The model under review builds one solid part; all positions refer to its coordinate system, in mm. A direction names the side the tool comes from. Round coordinates to 2 decimals unless told otherwise and drop trailing zeros. Loops run counter-clockwise (first coordinate to the right, second up) from the corner with the lowest first, then second, coordinate; pieces in that order, holes last. Notation, with made-up numbers: M -26,-11 L 23,-11 A23 cw 23,6 Z; hole C -39.75,-34 d7. An arc over 180 degrees is marked long. Return JSON: item names as keys, results as strings. Group by question number.
Q1. Consider section C-C (x = 15.5). State the section outline as (y, z) points (3 decimals).
Q2. Consider section D-D (y = -28). Count the separate pieces of the cut face and the enclosed holes in it, and give its area (3 significant figures).
Q3. Draft analysis for pull direction Y (two halves, no side actions). For faces 1 (the face through (0, -5, -54)), 2 (the face through (15.697, -55.431, 42.503)), 3 (the face through (16, -9.525, 24)), state which applies: pulls with the +Y half, pulls with the -Y half, needs draft (parallel to the pull), parting line crosses it, or undercut.
Q4. Consider section A-A (z = 0). State the section outline as (x, y) points (3 decimals), and give its area (3 significant figures).
Q5. To check wall thickness, follow line 1 along Y through (x, z) = (23, 18) (3 decimals); line 2 along Y through (x, z) = (24.5, 17) (3 decimals); line 3 along Z through (x, y) = (7, 19) (3 decimals). State the ranges of each line that lie inside material, in increasing order.
Q6. Clearance check with flat-ended pins moving along their axes: pin 1 Ø15 at (x, y) = (14.5, -29) entering from -Z; pin 2 Ø5.5 at (x, y) = (11.5, 27) entering from -Z; pin 3 Ø5 at (x, z) = (11.5, -40) entering from -Y. State where each tip first meets the part, or that it passes through.
Q7. For faces 4 (the face through (27.01, -49.592, 11.012)), 5 (the face through (16.01, 10.43, 10.48)), 6 (the face through (31.75, -5, -54)), list the 3-axis set-ups (+Z, -Z, +X, -X, +Y, -Y) from which the entire face can be reached by the end or side of a thin tool; tool diameter is ignored.
Autodesk Inventor part; units mm, degrees
ref_plane "YZ Plane" through (0, 0, 0) normal (1, 0, 0) x (0, 1, 0)
ref_plane "XZ Plane" through (0, 0, 0) normal (0, 1, 0) x (-1, 0, 0)
ref_plane "XY Plane" through (0, 0, 0) normal (0, 0, 1) x (1, 0, 0)
sketch "Sketch1" plane through (0, 0, 0) normal (1, 0, 0) x (0, 1, 0)
  point P0 (0, 0)
sketch "Sketch2" plane through (0, 0, 0) normal (1, 0, 0) x (0, 1, 0)
  circle A0 centre (0, 0) radius 69.85
  dimension "d0" = 139.7
extrude "Extrusion1" add sketch "Sketch2" along normal blind 31.75
sketch "Sketch3" plane through (0, 0, 0) normal (-1, 0, 0) x (0, 0, 1)
  circle A0 centre (0, 0) radius 50.8
  dimension "d3" = 101.6
extrude "Extrusion2" cut sketch "Sketch3" against normal blind 6.35
sketch "Sketch4" plane through (31.75, 0, 0) normal (1, 0, 0) x (0, 0, -1)
  circle A0 centre (0, 0) radius 50.8
  dimension "d6" = 101.6
extrude "Extrusion3" cut sketch "Sketch4" against normal blind 6.35
sketch "Sketch5" plane through (6.35, 0, 0) normal (-1, 0, 0) x (0, 0, 1)
  circle A0 centre (0, 0) radius 9.525
  line L0 (9.525, 0) -> (9.525, 40.1609)
  circle A1 centre (0, 0) radius 50.8
  line L1 (9.525, -9.525) -> (9.525, -40.1609)
  line L2 (-9.525, 9.525) -> (-40.1609, 9.525)
  line L3 (9.525, 9.525) -> (40.1609, 9.525)
  line L4 (-9.525, 9.525) -> (-9.525, 40.1609)
  line L5 (-9.525, -9.525) -> (-9.525, -40.1609)
  line L6 (-9.525, -9.525) -> (-40.1609, -9.525)
  line L7 (9.525, -9.525) -> (40.1609, -9.525)
  arc A2 (9.525, -40.1609) -> (40.1609, -9.525) centre (0, 0) ccw
  arc A3 (40.1609, 9.525) -> (9.525, 40.1609) centre (0, 0) ccw
  arc A4 (-9.525, 40.1609) -> (-40.1609, 9.525) centre (0, 0) ccw
  arc A5 (-40.1609, -9.525) -> (-9.525, -40.1609) centre (0, 0) ccw
sketch "Sketch6" plane through (6.35, 0, 0) normal (-1, 0, 0) x (0, 0, 1)
  point P0 (0, 0)
sketch "Sketch7" plane through (6.35, 0, 0) normal (-1, 0, 0) x (0, 0, 1)
  point P0 (0, 0)
extrude "Extrusion4" cut sketch "Sketch5" against normal through all contours A0 | L0 A3 L3 | L7 A2 L1 | L2 A4 L4 | L5 A5 L6
fillet "Fillet1" radius 3.175 12 edges at (15.875, 9.525, -9.525) (15.875, 9.525, 9.525) (15.875, -9.525, 9.525) (15.875, 40.1609, 9.525) (15.875, 9.525, 40.1609) (15.875, -40.1609, 9.525) (15.875, 9.525, -40.1609) (15.875, -9.525, -9.525) (15.875, -9.525, -40.1609) (15.875, -40.1609, -9.525) (15.875, -9.525, 40.1609) (15.875, 40.1609, -9.525)
fillet "Fillet2" radius 3.175 4 edges at (0, -69.85, 0) (0, 0, -50.8) (31.75, -69.85, 0) (31.75, 0, 50.8)
sketch "Sketch8" plane through (31.75, 0, 0) normal (1, 0, 0) x (0, 0, -1)
  point P0 (0, 0)
sketch "Sketch9" plane through (0, 0, 0) normal (0, 1, 0) x (-1, 0, 0)
  point P0 (0, 0)
sketch "Sketch10" plane through (25.4, 0, 0) normal (1, 0, 0) x (0, 0, -1)
  point P0 (0, 0)
properties part number "cock wheel"
Values:
{
 "1": {"outline": "C 0,0 d139.7; hole M -38.914,-13.758 A41.275 ccw -13.758,-38.914 A3.175 ccw -9.525,-35.921 L -9.525,-12.7 A3.175 ccw -12.7,-9.525 L -35.921,-9.525 A3.175 ccw Z; hole M -38.914,13.758 A3.175 ccw -35.921,9.525 L -12.7,9.525 A3.175 ccw -9.525,12.7 L -9.525,35.921 A3.175 ccw -13.758,38.914 A41.275 ccw Z; hole C 0,0 d19.05; hole M 9.525,-35.921 A3.175 ccw 13.758,-38.914 A41.275 ccw 38.914,-13.758 A3.175 ccw 35.921,-9.525 L 12.7,-9.525 A3.175 ccw 9.525,-12.7 Z; hole M 9.525,12.7 A3.175 ccw 12.7,9.525 L 35.921,9.525 A3.175 ccw 38.914,13.758 A41.275 ccw 13.758,38.914 A3.175 ccw 9.525,35.921 Z"},
 "2": {"separate pieces": "3", "enclosed holes": "0", "area": "2,170 mm2"},
 "3": {"face 1": "needs draft", "face 2": "parting line crosses it", "face 3": "undercut"},
 "4": {"outline": "M 0,-66.675 A3.175 ccw 3.175,-69.85 L 28.575,-69.85 A3.175 ccw 31.75,-66.675 L 31.75,-53.975 A3.175 ccw 28.575,-50.8 L 25.4,-50.8 L 25.4,-9.525 L 6.35,-9.525 L 6.35,-50.8 L 3.175,-50.8 A3.175 ccw 0,-53.975 Z; M 0,53.975 A3.175 ccw 3.175,50.8 L 6.35,50.8 L 6.35,9.525 L 25.4,9.525 L 25.4,50.8 L 28.575,50.8 A3.175 ccw 31.75,53.975 L 31.75,66.675 A3.175 ccw 28.575,69.85 L 3.175,69.85 A3.175 ccw 0,66.675 Z", "area": "2,760 mm2"},
 "5": {"line 1": "y = -67.491 to -37.143, -9.525 to 9.525, 37.143 to 67.491", "line 2": "y = -67.75 to -37.611, -9.525 to 9.525, 37.611 to 67.75", "line 3": "z = -67.216 to -36.642, -9.525 to 9.525, 36.642 to 67.216"},
 "6": {"pin 1": "stops at z = -66.46", "pin 2": "stops at z = -65.51", "pin 3": "stops at y = -58.93"},
 "7": {"face 4": "+X", "face 5": "+X, -X", "face 6": "+Z, -Z, +X, +Y, -Y"}
}
